Autodesk Inventor part; units mm, degrees
ref_plane "YZ Plane" through (0, 0, 0) normal (1, 0, 0) x (0, 1, 0)
ref_plane "XZ Plane" through (0, 0, 0) normal (0, 1, 0) x (-1, 0, 0)
ref_plane "XY Plane" through (0, 0, 0) normal (0, 0, 1) x (1, 0, 0)
sketch "スケッチ1" plane through (0, 0, 0) normal (0, 1, 0) x (-1, 0, 0)
  line L0 (-300, 280) -> (300, 280)
  line L1 (300, 280) -> (300, -280)
  line L2 (300, -280) -> (-300, -280)
  line L3 (-300, -280) -> (-300, 280)
  line L4 (-300, 280) -> (300, -280) construction
  line L5 (300, 280) -> (-300, -280) construction
  point P0 (0, 0)
  dimension "d0" = 600
  dimension "d1" = 560
extrude "押し出し1" add sketch "スケッチ1" along normal mid plane 6
sketch "スケッチ3" plane through (0, -3, 0) normal (0, -1, 0) x (1, 0, 0)
  circle A0 centre (-40, 115) radius 2.5
  line L0 (300, -280) -> (300, 280)
  line L1 (-300, -280) -> (300, -280)
  circle A1 centre (-140, 185) radius 2.5
  circle A2 centre (280, 40) radius 2.5
  point P0 (0, 0)
  dimension "d10" = 5
  dimension "d15" = 5
  dimension "d16" = 320
  dimension "d17" = 20
  dimension "d18" = 5
  dimension "d24" = 75
  dimension "d25" = 320
  dimension "d26" = 420
  dimension "d27" = 145
extrude "押し出し4" cut sketch "スケッチ3" against normal through all
sketch "スケッチ5" plane through (0, -3, 0) normal (0, -1, 0) x (1, 0, 0)
  line L0 (300, 250) -> (-300, 250)
  line L1 (-250, 280) -> (-250, -280) construction
  line L2 (-300, -250) -> (300, -250)
  line L3 (250, -280) -> (250, 280) construction
  line L4 (-300, 280) -> (300, 280)
  line L5 (-150, 280) -> (300, 120)
  line L6 (300, 280) -> (300, -280)
  line L7 (-300, -280) -> (-300, 280)
  line L8 (-300, 120) -> (-144.115427, -150)
  line L9 (-144.115427, -150) -> (300, -150)
  line L10 (300, -280) -> (300, 280)
  point P0 (0, 0)
  dimension "d32" = 100
  dimension "d33" = 130
  dimension "d34" = 400
  dimension "d35" = 60
  dimension "d46" = 270
sketch "スケッチ5 outline for 押し出し5" plane through (0, -3, 0) normal (0, -1, 0) x (1, 0, 0)
  line L0 (300, 120) -> (300, 280)
  line L1 (-150, 280) -> (300, 120)
  line L2 (300, 280) -> (-150, 280)
  line L3 (-300, 120) -> (-300, -280)
  line L4 (-144.115427, -150) -> (-300, 120)
  line L5 (300, -150) -> (-144.115427, -150)
  line L6 (300, -280) -> (300, -150)
  line L7 (-300, -280) -> (300, -280)
extrude "押し出し5" cut sketch "スケッチ5 outline for 押し出し5" against normal through all
chamfer "面取り2" distance 170 distance2 100 1 edges at (-144.1154, 0, -150) measured on face at (151.9615, -1, -150)
properties part number "endplate" material "CFRP"
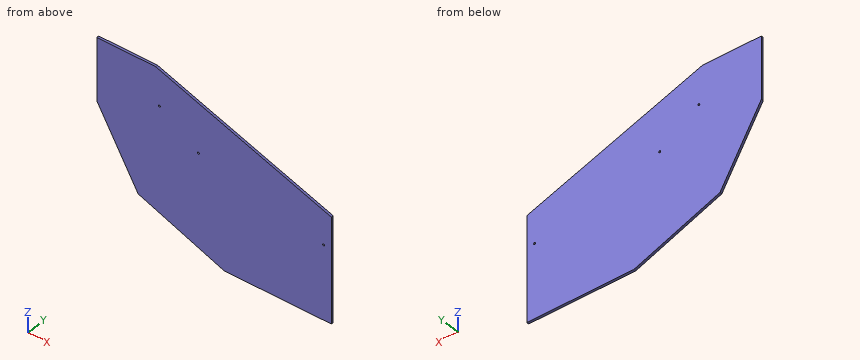
The listing builds one solid part. Answer for the finished solid, in the listing's coordinates (mm). Coordinates: 2 decimals unless noted, no trailing zeros. Loops run counter-clockwise (first coordinate to the right, second up) from the corner with the lowest first, then second, coordinate; pieces in that order, holes last. Notation, with made-up numbers: (88, -37.5) -> (126, -37.5) arc R34 ccw to (126, -7.5) -> close; hole circle Ø10 at (19.5, -25). An arc over 180 degrees is marked (long way). Return JSON: item names as keys, results as strings. Group by question number.
(1) A cutting plane is placed at C-C on x = -122. Write down the section's boundary in (y, z).
(2) A cutting plane is placed at A-A on y = -1.95. Write down the section's boundary in (x, z), and give its area (3 significant figures).
(3) A cutting plane is placed at B-B on z = 240. Write down the section's boundary in (x, y).
(4) Find the intervals of material crossed by probe 1 along Z at (x, y) = (-140, -0.3); probe 2 along Z at (x, y) = (280, 1.3); probe 3 along X at (y, z) = (-1.25, 48), in increasing order. Write a range as from..to.
(5) Given pin 1 Ø3 at (x, y) = (82.5, 0) entering from +Z; pin 2 Ø4.5 at (x, z) = (280, 40) entering from +Y; pin 3 Ø3 at (y, z) = (0.5, 70) entering from -X, each flat-ended and moving along its own axis, determine where each tip first touches the part or whether it passes through.
The answers:
{
 "1": {"outline": "(-3, -91.79) -> (3, -91.79) -> (3, 270.04) -> (-3, 270.04) -> close"},
 "2": {"outline": "(-300, 120) -> (-194.12, -63.4) -> (25.88, -150) -> (300, -150) -> (300, 120) -> (-150, 280) -> (-300, 280) -> close; hole circle Ø5 at (-140, 185); hole circle Ø5 at (-40, 115); hole circle Ø5 at (280, 40)", "area": "194,000 mm^2"},
 "3": {"outline": "(-300, -3) -> (-37.5, -3) -> (-37.5, 3) -> (-300, 3) -> close"},
 "4": {"probe 1": "z = -84.7..182.5, 187.5..276.44", "probe 2": "z = -150..37.5, 42.5..127.11", "probe 3": "x = -258.43..300"},
 "5": {"pin 1": "stops at z = 197.87", "pin 2": "passes through", "pin 3": "stops at x = -272"}
}
